Check sheet for the drawn part. Datum: minimum x, y, z corner. Units: mm. A direction names the side the tool comes from. Round coordinates to 2 decimals unless told otherwise and drop trailing zeros. Order: outer loops, then holes, each group sorted by start corner. A loop starts at its lowest first (then second) coordinate and runs counter-clockwise, first axis right, second up. Notation, with made-up numbers: (76.25, -26.5) -> (88.25, -26.5) arc R30 ccw to (88.25, 0.5) -> close; hole circle Ø4 at (25, 70). An arc over 180 degrees is marked (long way). Answer as a JSON object with one key per item and string values. Group by question number.
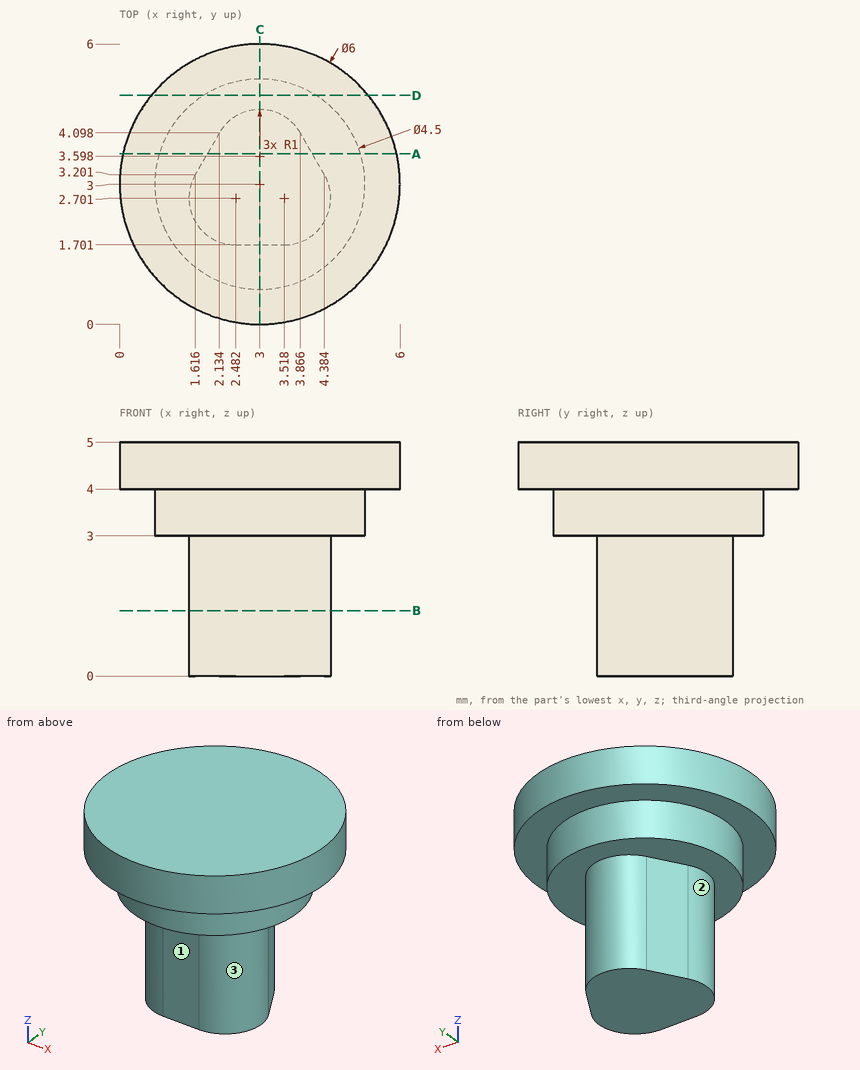
Item 1: Set-up check for the marked faces 1, 2 and 3: record each of +Z, -Z, +X, -X, +Y, -Y from which the full face is reachable in a straight line by a thin tool's end or side.
Item 2: Thickness scan on L1, parallel to Z at x = 4.55, y = 4.8; L2, parallel to Z at x = 3.5, y = 1.25; L3, parallel to Y at x = 3.05, z = 1.5. Record the ranges inside material, lowest first.
Item 3: Sectioned sample at B-B, the plane z = 1.4. Enter the section's corners in (x, y).
Item 4: Depth check by flat-ended pin: pin 1 Ø1.1 at (x, z) = (3, 2) entering from -Y; pin 2 Ø1 at (y, z) = (5.5, 4.5) entering from +X; pin 3 Ø2 at (y, z) = (2.5, 1.5) entering from +X. Enter the tip coordinate at first touch or a pass-through.
Item 5: Sectioned sample at D-D, the plane y = 4.9. Enter the section's corners in (x, z).
Item 6: Sectioned sample at C-C, the plane x = 3. Enter the section's corners in (y, z), then the cut area to 3 significant figures.
Item 7: Sectioned sample at A-A, the plane y = 3.65. Enter the section's corners in (x, z).
Result:
{
 "1": {"face 1": "-Z, +X, -X, -Y", "face 2": "-Z, -X", "face 3": "-Z, +X"},
 "2": {"L1": "z = 4 to 5", "L2": "z = 3 to 5", "L3": "y = 1.7 to 4.6"},
 "3": {"outline": "(1.62, 3.2) arc R1 ccw to (2.48, 1.7) -> (3.52, 1.7) arc R1 ccw to (4.38, 3.2) -> (3.87, 4.1) arc R1 ccw to (2.13, 4.1) -> close"},
 "4": {"pin 1": "stops at y = 1.7", "pin 2": "stops at x = 5.24", "pin 3": "stops at x = 4.52"},
 "5": {"outline": "(0.68, 4) -> (1.79, 4) -> (1.79, 3) -> (4.21, 3) -> (4.21, 4) -> (5.32, 4) -> (5.32, 5) -> (0.68, 5) -> close"},
 "6": {"outline": "(0, 4) -> (0.75, 4) -> (0.75, 3) -> (1.7, 3) -> (1.7, 0) -> (4.6, 0) -> (4.6, 3) -> (5.25, 3) -> (5.25, 4) -> (6, 4) -> (6, 5) -> (0, 5) -> close", "area": "19.2 mm2"},
 "7": {"outline": "(0.07, 4) -> (0.85, 4) -> (0.85, 3) -> (1.88, 3) -> (1.88, 0) -> (4.12, 0) -> (4.12, 3) -> (5.15, 3) -> (5.15, 4) -> (5.93, 4) -> (5.93, 5) -> (0.07, 5) -> close"}
}
